from build123d import *

# Parameters (mm, degrees)
SKETCH_R          = 15
SKETCH_R_2        = 7.5
PAD_DEPTH         = 20
SKETCH001_R       = 15
SKETCH001_R_2     = 4.5
PAD001_DEPTH      = 20
SKETCH002_W       = 20
SKETCH002_H       = 7
POCKET_DEPTH      = 40
POCKET_FACE2_W    = 1.18034
POCKET_FACE2_H    = 40
POCKET001_DEPTH   = 5
POCKET001_FACE2_W = 1.18034
POCKET001_FACE2_H = 40
POCKET002_DEPTH   = 5
POCKET002_FACE7_W = 22.36068
POCKET002_FACE7_H = 40
PAD002_DEPTH      = 5
FILLET_R          = 5
SKETCH003_R       = 2
POCKET003_DEPTH   = 13


with BuildPart() as part:
    # Sketch → Pad (new body)
    with BuildSketch(Plane.XY):
        Circle(SKETCH_R)
        Circle(SKETCH_R_2, mode=Mode.SUBTRACT)
    extrude(amount=PAD_DEPTH)

    # Sketch001 (on Face4 of Pad) → Pad001 (join)
    with BuildSketch(Plane.XY.offset(20)):
        Circle(SKETCH001_R)
        Circle(SKETCH001_R_2, mode=Mode.SUBTRACT)
    extrude(amount=PAD001_DEPTH)

    # Sketch002 (on Face1 of Pad001) → Pocket (cut)
    with BuildSketch(Plane(origin=(0, 0, 0), x_dir=(1, 0, 0), z_dir=(0, 0, -1))):
        with Locations((0, 13.5)):
            Rectangle(SKETCH002_W, SKETCH002_H)
    extrude(amount=-POCKET_DEPTH, mode=Mode.SUBTRACT)

    # Pocket Face2 → Pocket001 (cut)
    with BuildSketch(Plane(origin=(10, -10.59017, 20), x_dir=(0, 1, 0), z_dir=(-1, 0, 0))):
        Rectangle(POCKET_FACE2_W, POCKET_FACE2_H)
    extrude(amount=-POCKET001_DEPTH, mode=Mode.SUBTRACT)

    # Pocket001 Face2 → Pocket002 (cut)
    with BuildSketch(Plane(origin=(-10, -10.59017, 20), x_dir=(0, -1, 0), z_dir=(1, 0, 0))):
        Rectangle(POCKET001_FACE2_W, POCKET001_FACE2_H)
    extrude(amount=-POCKET002_DEPTH, mode=Mode.SUBTRACT)

    # Pocket002 Face7 → Pad002 (add)
    with BuildSketch(Plane(origin=(0, -10, 20), x_dir=(-1, 0, 0), z_dir=(0, -1, 0))):
        Rectangle(POCKET002_FACE7_W, POCKET002_FACE7_H)
    extrude(amount=PAD002_DEPTH)

    # Fillet
    fillet_edges = [part.edges().sort_by_distance(p)[0] for p in [
        (11.18034, -10, 20),
        (-11.18034, -10, 20),
    ]]
    fillet(fillet_edges, radius=FILLET_R)

    # Sketch003 (on Face7 of Fillet) → Pocket003 (cut)
    with BuildSketch(Plane.XZ.offset(15)):
        with Locations((0, 35)):
            Circle(SKETCH003_R)
        with Locations((0, 14)):
            Circle(SKETCH003_R)
        with Locations((0, 28)):
            Circle(SKETCH003_R)
        with Locations((0, 7)):
            Circle(SKETCH003_R)
    extrude(amount=-POCKET003_DEPTH, mode=Mode.SUBTRACT)


solid = part.part
Verification items for the finished model (mm, model axes). A direction names the side the tool comes from. Coordinates: 2 decimals unless noted, no trailing zeros. Order: outer loops, then holes, each group sorted by start corner. A loop starts at its lowest first (then second) coordinate and runs counter-clockwise, first axis right, second up. Notation, with made-up numbers: M 83.25,39 L 133.25,39 A18 cw 133.25,67 Z; hole C 27,81.5 d6. An arc over 180 degrees is marked long. Return JSON: item names as keys, results as strings.
1) Cross-section at C-C, the plane x = 0. Record the boundary of the cut face in (y, z).
Answer list:
{"outline": "M -15,0 L -7.5,0 L -7.5,5 L -15,5 Z; M -15,9 L -7.5,9 L -7.5,12 L -15,12 Z; M -15,16 L -7.5,16 L -7.5,20 L -4.5,20 L -4.5,26 L -15,26 Z; M -15,30 L -4.5,30 L -4.5,33 L -15,33 Z; M -15,37 L -4.5,37 L -4.5,40 L -15,40 Z; M 4.5,20 L 7.5,20 L 7.5,0 L 15,0 L 15,40 L 4.5,40 Z"}
2) Access from +Z, -Z, +X, -X, +Y, -Y to the whole of each face (thin tool, end or side, straight path). Record for faces 1 (the flat face through (11.18, -13, 20)), 2 (the flat face through (-11.18, -13, 20)), 3 (the cylindrical face through (0, -10, 26)), 4 (the cylindrical face through (-0.976, 7.436, 9.86)).
Answer list:
{"face 1": "+Z, -Z, +X, -Y", "face 2": "+Z, -Z, -X, -Y", "face 3": "-Y", "face 4": "-Z"}
3) Cross-section at B-B, the plane z = 11. Record the boundary of the cut face in (x, y).
Answer list:
{"outline": "M -12.14,-8.82 A5 cw -11.18,-11.76 L -11.18,-15 L 11.18,-15 L 11.18,-11.76 A5 cw 12.14,-8.82 A15 ccw long Z; hole C 0,0 d15"}
4) Cross-section at D-D, the plane z = 25.5. Record the boundary of the cut face in (x, y), and give its area (3 significant figures).
Answer list:
{"outline": "M -12.14,-8.82 A5 cw -11.18,-11.76 L -11.18,-15 L 11.18,-15 L 11.18,-11.76 A5 cw 12.14,-8.82 A15 ccw long Z; hole C 0,0 d9", "area": "678 mm2"}
5) Gauge pin test, flat ends, axial feed: pin 1 (12 mm diameter, centred on x = 0, y = 0, fed in from -Z); pin 2 (5 mm diameter, centred on y = -5, z = 15, fed in from +X); pin 3 (3.5 mm diameter, centred on y = -13.5, z = 19, fed in from -X). Record the tip position at first contact, or that the pin passes through.
Answer list:
{"pin 1": "z = 20", "pin 2": "x = 14.79", "pin 3": "x = -11.18"}
6) Release check for a two-part mould opening along Z. For faces 5 (the cylindrical face through (0, -10, 33)), 6 (the cylindrical face through (0, -11, 9)), 7 (the flat face through (4, -3, 40)), 8 (the cylindrical face through (0, 15, 20)) record: +Z half, -Z half, draft (parallel to the pull), parting line (faces both ways), or undercut.
Answer list:
{"face 5": "undercut", "face 6": "undercut", "face 7": "+Z half", "face 8": "draft"}
7) Cross-section at A-A, the plane y = 0. Record the boundary of the cut face in (x, z).
Answer list:
{"outline": "M -15,0 L -7.5,0 L -7.5,20 L -4.5,20 L -4.5,40 L -15,40 Z; M 4.5,20 L 7.5,20 L 7.5,0 L 15,0 L 15,40 L 4.5,40 Z"}
8) Thickness scan on L1, parallel to Z at x = 0, y = -12.25; L2, parallel to Y at x = -0.25, z = 4; L3, parallel to X at y = -12, z = 28. Record the ranges inside material, lowest first. Write a range as [from, to].
Answer list:
{"L1": "[0, 5], [9, 12], [16, 26], [30, 33], [37, 40]", "L2": "[-15, -7.5], [7.5, 15]", "L3": "[-11.18, -2], [2, 11.18]"}
